```python
from build123d import *

# Parameters (mm, degrees)
F0_R     = 55.750000441
F0_R_2   = 49.75
F1_DEPTH = 13
F3_R     = 5
F4_DEPTH = 10
F5_SIZE2 = 2.292241
F5_SIZE  = 12.99999
F6_SIZE2 = 5
F6_SIZE  = 1


# Not quite as in the source:
# - a fillet or chamfer is up to 0.001 mm smaller than in the source, because OpenCascade refuses the exact size


with BuildPart() as f1:
    # F0 (on Top) → F1 (new body)
    with BuildSketch(Plane.XY):
        Circle(F0_R)
        Circle(F0_R_2, mode=Mode.SUBTRACT)
    extrude(amount=F1_DEPTH)

    # F3 (on offset) → F4 (join)
    with BuildSketch(Plane.XZ.offset(54)):
        with Locations((0, 6.4556576599)):
            Circle(F3_R)
    extrude(amount=F4_DEPTH)

    # F5 (size 13 and 2.2922507492 in the source; OpenCascade refuses exactly that, so slightly less here)
    f5_edges = [f1.edges().sort_by_distance(p)[0] for p in [
        (-49.75, 0, 13),
    ]]
    f5_side = f1.faces().sort_by_distance((-49.75, 0, 6.5))[0]
    chamfer(f5_edges, length=F5_SIZE, length2=F5_SIZE2, reference=f5_side)

    # F6
    f6_edges = [f1.edges().sort_by_distance(p)[0] for p in [
        (-5, -64, 6.455658),
    ]]
    f6_side = f1.faces().sort_by_distance((0, -64, 6.455658))[0]
    chamfer(f6_edges, length=F6_SIZE, length2=F6_SIZE2, reference=f6_side)


solid = f1.part
```
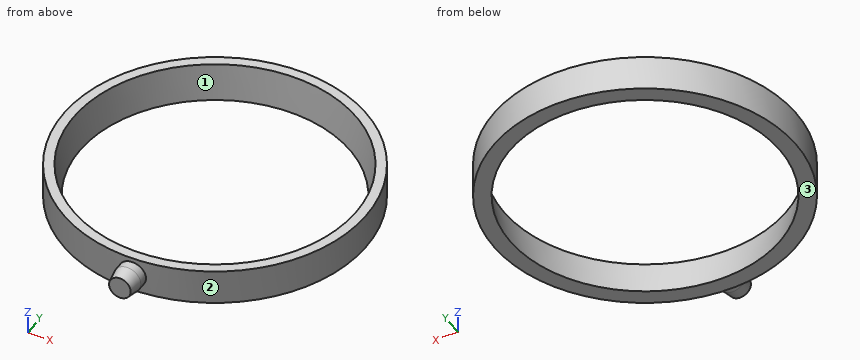
Here's how the part is built. I have some questions about the finished solid (model axes, mm). Face numbers are marked on the shaded views. Round coordinates to 2 decimals unless told otherwise and drop trailing zeros.
Q1. If we mould it in two halves opening along X, with no side actions, what happens to the marked faces 1, 2 and 3? For each: +X half, -X half, draft (parallel to the pull), parting line (faces both ways), or undercut.
Q2. Please list where these lines run through material, in increasing order: probe 1 along Y at (x, z) = (0, 0.05); probe 2 along X at (y, z) = (-41.5, 9); probe 3 along X at (y, z) = (-42.5, 2.5).
Q3. Will these pins go through, and if not, where does the flat tip stop? P1, Ø1, axis at x = -31.5, z = 10, coming from the -Y side; P2, Ø3, axis at x = -3.5, z = 7, coming from the +Y side; P3, Ø1.5, axis at x = 41.5, z = 7, coming from the +Y side.
Answer below:
1. face 1: undercut
1. face 2: parting line
1. face 3: draft
2. probe 1: y = -55.75 to -49.76, 49.76 to 55.75
2. probe 2: x = -37.23 to -30.22, 30.22 to 37.23
2. probe 3: x = -36.08 to -26.7, 26.7 to 36.08
3. P1: stops at y = -46.34
3. P2: stops at y = 55.71
3. P3: stops at y = 38.05
